The listing builds one solid part. Answer for the finished solid, in the listing's coordinates (mm). A direction names the side the tool comes from. Coordinates: 2 decimals unless noted, no trailing zeros. Write each loop counter-clockwise with the first axis right and the second up, starting at its lowest first coordinate (ties: lowest second). Pieces come first, ordered by that corner, then holes. Notation, with made-up numbers: M 24,9 L 82,9 A27 cw 82,46 Z; hole C 67,-32 d4. An arc over 180 degrees is marked long. Write item = value, one per line. Start each with the question number.
```python
from build123d import *

# Parameters (mm, degrees)
F0_R         = 11.1
F1_DEPTH     = 6
F2_C1_SIZE2  = 3
F2_C1_SIZE   = 1.7320508076
F2_C2_SIZE2  = 3
F2_C2_SIZE   = 1.7320508076
F2_C3_SIZE2  = 3
F2_C3_SIZE   = 1.7320508076
F2_C4_SIZE2  = 3
F2_C4_SIZE   = 1.7320508076
F2_C5_SIZE2  = 1.7320508076
F2_C5_SIZE   = 3
F2_C6_SIZE2  = 3
F2_C6_SIZE   = 1.7320508076
F2_C7_SIZE2  = 1.7320508076
F2_C7_SIZE   = 3
F2_C8_SIZE2  = 3
F2_C8_SIZE   = 1.7320508076
F2_C9_SIZE2  = 1.7320508076
F2_C9_SIZE   = 3
F2_C10_SIZE2 = 3
F2_C10_SIZE  = 1.7320508076
F2_C11_SIZE2 = 3
F2_C11_SIZE  = 1.7320508076
F2_C12_SIZE2 = 3
F2_C12_SIZE  = 1.7320508076
F2_C13_SIZE2 = 1.7320508076
F2_C13_SIZE  = 3
F2_C14_SIZE2 = 3
F2_C14_SIZE  = 1.7320508076
F2_C15_SIZE2 = 3
F2_C15_SIZE  = 1.7320508076
F2_C16_SIZE2 = 3
F2_C16_SIZE  = 1.7320508076
F2_C17_SIZE2 = 1.7320508076
F2_C17_SIZE  = 3
F2_C18_SIZE2 = 3
F2_C18_SIZE  = 1.7320508076
F2_C19_SIZE2 = 3
F2_C19_SIZE  = 1.7320508076
F2_C20_SIZE2 = 3
F2_C20_SIZE  = 1.7320508076
F2_C21_SIZE2 = 1.7320508076
F2_C21_SIZE  = 3
F2_C22_SIZE2 = 3
F2_C22_SIZE  = 1.7320508076
F2_C23_SIZE2 = 3
F2_C23_SIZE  = 1.7320508076
F2_C24_SIZE2 = 3
F2_C24_SIZE  = 1.7320508076
F3_R         = 0.875


with BuildPart() as f1:
    # F0 (on Top) → F1 (new body)
    with BuildSketch(Plane.XY):
        with BuildLine():
            Line((8.3388454559, 22.1051900243), (0, 45))
            Line((0, 45), (-8.3388454559, 22.1051900243))
            ThreePointArc((-8.3388454559, 22.1051900243), (-7.55, 13.0769835971), (-14.9742333886, 18.2742470152))
            Line((-14.9742333886, 18.2742470152), (-38.9711431703, 22.5))
            Line((-38.9711431703, 22.5), (-23.3130788445, 3.8309430091))
            ThreePointArc((-23.3130788445, 3.8309430091), (-15.1, 0), (-23.3130788445, -3.8309430091))
            Line((-23.3130788445, -3.8309430091), (-38.9711431703, -22.5))
            Line((-38.9711431703, -22.5), (-14.9742333886, -18.2742470152))
            ThreePointArc((-14.9742333886, -18.2742470152), (-7.55, -13.0769835971), (-8.3388454559, -22.1051900243))
            Line((-8.3388454559, -22.1051900243), (0, -45))
            Line((0, -45), (8.3388454559, -22.1051900243))
            ThreePointArc((8.3388454559, -22.1051900243), (7.55, -13.0769835971), (14.9742333886, -18.2742470152))
            Line((14.9742333886, -18.2742470152), (38.9711431703, -22.5))
            Line((38.9711431703, -22.5), (23.3130788445, -3.8309430091))
            ThreePointArc((23.3130788445, -3.8309430091), (15.1, 0), (23.3130788445, 3.8309430091))
            Line((23.3130788445, 3.8309430091), (38.9711431703, 22.5))
            Line((38.9711431703, 22.5), (14.9742333886, 18.2742470152))
            ThreePointArc((14.9742333886, 18.2742470152), (7.55, 13.0769835971), (8.3388454559, 22.1051900243))
        make_face()
        Circle(F0_R, mode=Mode.SUBTRACT)
    extrude(amount=F1_DEPTH)

    # F2: chamfer of 3 x 1.7320508076 on 24 edges, made by hand

    # F2_c1
    f2_c1_edges = [f1.edges().sort_by_distance(p)[0] for p in [
        (31.1421110074, 13.1654715045, 0),
    ]]
    f2_c1_side = f1.faces().sort_by_distance((31.1421110074, 13.1654715045, 0.0346410162))[0]
    chamfer(f2_c1_edges, length=F2_C1_SIZE, length2=F2_C1_SIZE2, reference=f2_c1_side)

    # F2_c2
    f2_c2_edges = [f1.edges().sort_by_distance(p)[0] for p in [
        (31.1421110074, 13.1654715045, 6),
    ]]
    f2_c2_side = f1.faces().sort_by_distance((31.1421110074, 13.1654715045, 5.9653589838))[0]
    chamfer(f2_c2_edges, length=F2_C2_SIZE, length2=F2_C2_SIZE2, reference=f2_c2_side)

    # F2_c3
    f2_c3_edges = [f1.edges().sort_by_distance(p)[0] for p in [
        (24.6756919125, 19.9826322901, 0),
    ]]
    f2_c3_side = f1.faces().sort_by_distance((24.6816996097, 19.9485162005, 0))[0]
    chamfer(f2_c3_edges, length=F2_C3_SIZE, length2=F2_C3_SIZE2, reference=f2_c3_side)

    # F2_c4
    f2_c4_edges = [f1.edges().sort_by_distance(p)[0] for p in [
        (24.6756919125, 19.9826322901, 6),
    ]]
    f2_c4_side = f1.faces().sort_by_distance((24.6756919125, 19.9826322901, 5.9653589838))[0]
    chamfer(f2_c4_edges, length=F2_C4_SIZE, length2=F2_C4_SIZE2, reference=f2_c4_side)

    # F2_c5
    f2_c5_edges = [f1.edges().sort_by_distance(p)[0] for p in [
        (4.169422728, 33.5525950122, 0),
    ]]
    f2_c5_side = f1.faces().sort_by_distance((4.136873479, 33.5407397857, 0))[0]
    chamfer(f2_c5_edges, length=F2_C5_SIZE, length2=F2_C5_SIZE2, reference=f2_c5_side)

    # F2_c6
    f2_c6_edges = [f1.edges().sort_by_distance(p)[0] for p in [
        (4.169422728, 33.5525950122, 6),
    ]]
    f2_c6_side = f1.faces().sort_by_distance((4.169422728, 33.5525950122, 5.9653589838))[0]
    chamfer(f2_c6_edges, length=F2_C6_SIZE, length2=F2_C6_SIZE2, reference=f2_c6_side)

    # F2_c7
    f2_c7_edges = [f1.edges().sort_by_distance(p)[0] for p in [
        (-4.9676212415, 31.3610921973, 0),
    ]]
    f2_c7_side = f1.faces().sort_by_distance((-4.9350719925, 31.3492369708, 0))[0]
    chamfer(f2_c7_edges, length=F2_C7_SIZE, length2=F2_C7_SIZE2, reference=f2_c7_side)

    # F2_c8
    f2_c8_edges = [f1.edges().sort_by_distance(p)[0] for p in [
        (-4.9676212415, 31.3610921973, 6),
    ]]
    f2_c8_side = f1.faces().sort_by_distance((-4.9676212415, 31.3610921973, 5.9653589838))[0]
    chamfer(f2_c8_edges, length=F2_C8_SIZE, length2=F2_C8_SIZE2, reference=f2_c8_side)

    # F2_c9
    f2_c9_edges = [f1.edges().sort_by_distance(p)[0] for p in [
        (-26.9726882794, 20.3871235076, 0),
    ]]
    f2_c9_side = f1.faces().sort_by_distance((-26.9786959766, 20.353007418, 0))[0]
    chamfer(f2_c9_edges, length=F2_C9_SIZE, length2=F2_C9_SIZE2, reference=f2_c9_side)

    # F2_c10
    f2_c10_edges = [f1.edges().sort_by_distance(p)[0] for p in [
        (-26.9726882794, 20.3871235076, 6),
    ]]
    f2_c10_side = f1.faces().sort_by_distance((-26.9726882794, 20.3871235076, 5.9653589838))[0]
    chamfer(f2_c10_edges, length=F2_C10_SIZE, length2=F2_C10_SIZE2, reference=f2_c10_side)

    # F2_c11
    f2_c11_edges = [f1.edges().sort_by_distance(p)[0] for p in [
        (-29.643313154, 11.3784599071, 0),
    ]]
    f2_c11_side = f1.faces().sort_by_distance((-29.6167716023, 11.4007207704, 0))[0]
    chamfer(f2_c11_edges, length=F2_C11_SIZE, length2=F2_C11_SIZE2, reference=f2_c11_side)

    # F2_c12
    f2_c12_edges = [f1.edges().sort_by_distance(p)[0] for p in [
        (-29.643313154, 11.3784599071, 6),
    ]]
    f2_c12_side = f1.faces().sort_by_distance((-29.643313154, 11.3784599071, 5.9653589838))[0]
    chamfer(f2_c12_edges, length=F2_C12_SIZE, length2=F2_C12_SIZE2, reference=f2_c12_side)

    # F2_c13
    f2_c13_edges = [f1.edges().sort_by_distance(p)[0] for p in [
        (-31.1421110074, -13.1654715045, 0),
    ]]
    f2_c13_side = f1.faces().sort_by_distance((-31.1155694557, -13.1877323678, 0))[0]
    chamfer(f2_c13_edges, length=F2_C13_SIZE, length2=F2_C13_SIZE2, reference=f2_c13_side)

    # F2_c14
    f2_c14_edges = [f1.edges().sort_by_distance(p)[0] for p in [
        (-31.1421110074, -13.1654715045, 6),
    ]]
    f2_c14_side = f1.faces().sort_by_distance((-31.1421110074, -13.1654715045, 5.9653589838))[0]
    chamfer(f2_c14_edges, length=F2_C14_SIZE, length2=F2_C14_SIZE2, reference=f2_c14_side)

    # F2_c15
    f2_c15_edges = [f1.edges().sort_by_distance(p)[0] for p in [
        (-24.6756919125, -19.9826322901, 0),
    ]]
    f2_c15_side = f1.faces().sort_by_distance((-24.6816996097, -19.9485162005, 0))[0]
    chamfer(f2_c15_edges, length=F2_C15_SIZE, length2=F2_C15_SIZE2, reference=f2_c15_side)

    # F2_c16
    f2_c16_edges = [f1.edges().sort_by_distance(p)[0] for p in [
        (-24.6756919125, -19.9826322901, 6),
    ]]
    f2_c16_side = f1.faces().sort_by_distance((-24.6756919125, -19.9826322901, 5.9653589838))[0]
    chamfer(f2_c16_edges, length=F2_C16_SIZE, length2=F2_C16_SIZE2, reference=f2_c16_side)

    # F2_c17
    f2_c17_edges = [f1.edges().sort_by_distance(p)[0] for p in [
        (-4.169422728, -33.5525950122, 0),
    ]]
    f2_c17_side = f1.faces().sort_by_distance((-4.136873479, -33.5407397857, 0))[0]
    chamfer(f2_c17_edges, length=F2_C17_SIZE, length2=F2_C17_SIZE2, reference=f2_c17_side)

    # F2_c18
    f2_c18_edges = [f1.edges().sort_by_distance(p)[0] for p in [
        (-4.169422728, -33.5525950122, 6),
    ]]
    f2_c18_side = f1.faces().sort_by_distance((-4.169422728, -33.5525950122, 5.9653589838))[0]
    chamfer(f2_c18_edges, length=F2_C18_SIZE, length2=F2_C18_SIZE2, reference=f2_c18_side)

    # F2_c19
    f2_c19_edges = [f1.edges().sort_by_distance(p)[0] for p in [
        (4.9676212415, -31.3610921973, 0),
    ]]
    f2_c19_side = f1.faces().sort_by_distance((4.9350719925, -31.3492369708, 0))[0]
    chamfer(f2_c19_edges, length=F2_C19_SIZE, length2=F2_C19_SIZE2, reference=f2_c19_side)

    # F2_c20
    f2_c20_edges = [f1.edges().sort_by_distance(p)[0] for p in [
        (4.9676212415, -31.3610921973, 6),
    ]]
    f2_c20_side = f1.faces().sort_by_distance((4.9676212415, -31.3610921973, 5.9653589838))[0]
    chamfer(f2_c20_edges, length=F2_C20_SIZE, length2=F2_C20_SIZE2, reference=f2_c20_side)

    # F2_c21
    f2_c21_edges = [f1.edges().sort_by_distance(p)[0] for p in [
        (26.9726882794, -20.3871235076, 0),
    ]]
    f2_c21_side = f1.faces().sort_by_distance((26.9786959766, -20.353007418, 0))[0]
    chamfer(f2_c21_edges, length=F2_C21_SIZE, length2=F2_C21_SIZE2, reference=f2_c21_side)

    # F2_c22
    f2_c22_edges = [f1.edges().sort_by_distance(p)[0] for p in [
        (26.9726882794, -20.3871235076, 6),
    ]]
    f2_c22_side = f1.faces().sort_by_distance((26.9726882794, -20.3871235076, 5.9653589838))[0]
    chamfer(f2_c22_edges, length=F2_C22_SIZE, length2=F2_C22_SIZE2, reference=f2_c22_side)

    # F2_c23
    f2_c23_edges = [f1.edges().sort_by_distance(p)[0] for p in [
        (29.643313154, -11.3784599071, 0),
    ]]
    f2_c23_side = f1.faces().sort_by_distance((29.6167716023, -11.4007207704, 0))[0]
    chamfer(f2_c23_edges, length=F2_C23_SIZE, length2=F2_C23_SIZE2, reference=f2_c23_side)

    # F2_c24
    f2_c24_edges = [f1.edges().sort_by_distance(p)[0] for p in [
        (29.643313154, -11.3784599071, 6),
    ]]
    f2_c24_side = f1.faces().sort_by_distance((29.643313154, -11.3784599071, 5.9653589838))[0]
    chamfer(f2_c24_edges, length=F2_C24_SIZE, length2=F2_C24_SIZE2, reference=f2_c24_side)

    # F3
    f3_edges = [f1.edges().sort_by_distance(p)[0] for p in [
        (-11.1, 0, 0),
        (-11.1, 0, 6),
    ]]
    fillet(f3_edges, radius=F3_R)


solid = f1.part
```
1. The part is cut by section B-B, the plane x = 27. Write down the section's boundary in (y, z).
2. The part is cut by section C-C, the plane y = 33.5. Write down the section's boundary in (x, z), and give its area (3 significant figures).
3. The part is cut by section D-D, the plane x = 16.5. Write down the section's boundary in (y, z), and give its area (3 significant figures).
4. For a pull along Y with two mould halves and no side action, classify faces 1 (the face through (-23.793, 18.283, 5.146)), 2 (the face through (-3, -12, 0)), 3 (the face through (31.252, -13.296, 3.625)) as pulls with the +Y half, pulls with the -Y half, needs draft (parallel to the pull), parting line crosses it, or undercut.
5. Each of these flat-tipped pins is pushed along its axis until it touches: pin 1 (3 mm diameter, centred on x = -26, y = 5, fed in from +Z); pin 2 (2 mm diameter, centred on y = 28, z = 3, fed in from +X); pin 3 (11.5 mm diameter, centred on x = -20.1, y = 0, fed in from -Z); pin 4 (2 mm diameter, centred on y = -26, z = 4.5, fed in from -X). Where does it stop, or does it pass through?
6. For faces 4 (the face through (30.5, -13.73, 1.52)), 5 (the face through (27.73, 11.464, 5.146)), 6 (the face through (-27.14, -19.55, 1.52)), determine the directions among +Z, -Z, +X, -X, +Y, -Y from which every point of the face is accessible in a straight line to the end or side of a thin tool.
7. The part is cut by section A-A, the plane y = 0. Write down the section's boundary in (x, z) (3 decimals).
8. Straight lines are drawn through the part: L1, parallel to X at y = -4, z = 4.25; L2, parallel to Y at x = 10.05, z = 4.05; L3, parallel to Y at x = 20, z = 5.5. For each, find the intervals that lie inside material, in ascending order. Write a range as [from, to].
Solution:
q1.outline = M -20.39,1.73 L -17.35,0 L -10.92,0 L -8.23,3 L -8.23,4.27 L -12.9,6 L -17.35,6 L -20.39,4.27 Z; M 8.23,1.73 L 12.9,0 L 18.63,0 L 20.39,3 L 20.39,4.27 L 17.35,6 L 12.9,6 L 8.23,4.27 Z
q2.outline = M -4.19,1.73 L -1,0 L 1,0 L 4.19,1.73 L 4.19,4.27 L 1,6 L -1,6 L -4.19,4.27 Z
q2.area = 39.2 mm^2
q3.outline = M -18.54,1.73 L -15.5,0 L -3.47,0 L -3.47,6 L -15.5,6 L -18.54,4.27 Z; M 3.47,0 L 16.78,0 L 18.54,3 L 18.54,4.27 L 15.5,6 L 3.47,6 Z
q3.area = 170 mm^2
q4.face_1 = pulls with the +Y half
q4.face_2 = needs draft
q4.face_3 = undercut
q5.pin_1 = 4.38
q5.pin_2 = 6.56
q5.pin_3 = 0
q5.pin_4 = -7.27
q6.face_4 = -Z, +X
q6.face_5 = +Z, +X
q6.face_6 = -Z, -Y
q7.outline = M -15.1,0 L -11.975,0 A0.875 ccw -11.1,0.875 L -11.1,5.125 A0.875 ccw -11.975,6 L -15.1,6 Z; M 11.1,0.875 A0.875 ccw 11.975,0 L 15.1,0 L 15.1,6 L 11.975,6 A0.875 ccw 11.1,5.125 Z
q8.L1 = [-23.45, -23.1], [-17.1, -10.35], [10.35, 17.1], [23.1, 23.45]
q8.L2 = [-12.41, -4.71], [4.71, 12.41]
q8.L3 = [-16.99, -5], [5, 16.99]
